from build123d import *

# Parameters (mm, degrees)
SKETCH3_R                = 3.571875
SKETCH3_R_2              = 1.5319375
SKETCH3_R_3              = 2.778125
SKETCH3_R_4              = 0.813693974
BOSS_EXTRUDE1_DEPTH      = 7.9375
BOSS_EXTRUDE2_DEPTH      = 9.525
BOSS_EXTRUDE2_DEPTH_BACK = 1.5875
SKETCH3_4_R              = 1.5319375
FILLET1_R                = 1.5875
SKETCH4_W                = 1.5875
SKETCH4_H                = 4.7625
CUT_EXTRUDE1_DEPTH       = 3.175
SKETCH5_W                = 4.7752
SKETCH5_H                = 1.5875
CUT_EXTRUDE2_DEPTH       = 3.175
FILLET2_R                = 3.571875
SKETCH6_R                = 0.4064
CUT_EXTRUDE4_DEPTH       = 0.89281
CUT_EXTRUDE6_START       = -1.5875
CUT_EXTRUDE6_DEPTH       = 1.5875
CUT_EXTRUDE7_START       = -7.9375
CUT_EXTRUDE7_DEPTH       = 1.5875
FILLET4_R                = 1.5875


with BuildPart() as part:
    # Sketch3 → Boss-Extrude1 (new body)
    # profile 1 of 12: a face of its own
    with BuildSketch(Plane.XY):
        with BuildLine():
            Line((11.069438658, 5.55625), (2.778125, 5.55625))
            ThreePointArc((2.778125, 5.55625), (4.742556026, 4.742556026), (5.55625, 2.778125))
            ThreePointArc((5.55625, 2.778125), (4.742556026, 0.813693974), (2.778125, 0))
            Line((2.778125, 0), (9.649461258, 0))
            ThreePointArc((9.649461258, 0), (10.438552252, 3.141997614), (13.44291972, 4.353851449))
            ThreePointArc((13.44291972, 4.353851449), (12.140043825, 4.7258047), (11.069438658, 5.55625))
        make_face()
    # profile 2 of 12: a face of its own
    with BuildSketch(Plane.XY):
        with Locations((13.754229109, 7.912134389)):
            Circle(SKETCH3_R)
        with Locations((13.754229109, 7.912134389)):
            Circle(SKETCH3_R_2, mode=Mode.SUBTRACT)
    # profile 3 of 12: a face of its own
    with BuildSketch(Plane.XY):
        with Locations((2.778125, 2.778125)):
            Circle(SKETCH3_R_3)
    # profile 4 of 12: a face of its own
    with BuildSketch(Plane.XY):
        with Locations((0.813693974, 4.742556026)):
            Circle(SKETCH3_R_4)
    # profile 5 of 12: a face of its own
    with BuildSketch(Plane.XY):
        with BuildLine():
            ThreePointArc((0.328789509, 4.089130022), (0.086830258, 4.376814286), (0, 4.742556026))
            Line((0, 4.742556026), (0, 2.778125))
            ThreePointArc((0, 2.778125), (0.083450745, 3.453927617), (0.328789509, 4.089130022))
        make_face()
    # profile 6 of 12: a face of its own
    with BuildSketch(Plane.XY):
        with Locations((2.778125, 2.778125)):
            Circle(SKETCH3_R_3)
    # profile 7 of 12: a face of its own
    with BuildSketch(Plane.XY):
        with Locations((0.813693974, 4.742556026)):
            Circle(SKETCH3_R_4)
    # profile 8 of 12: a face of its own
    with BuildSketch(Plane.XY):
        with Locations((0.813693974, 4.742556026)):
            Circle(SKETCH3_R_4)
    # profile 9 of 12: a face of its own
    with BuildSketch(Plane.XY):
        with Locations((2.778125, 2.778125)):
            Circle(SKETCH3_R_3)
    # profile 10 of 12: a face of its own
    with BuildSketch(Plane.XY):
        with BuildLine():
            Line((2.778125, 5.55625), (0.813693974, 5.55625))
            ThreePointArc((0.813693974, 5.55625), (1.179435714, 5.469419742), (1.467119978, 5.227460491))
            ThreePointArc((1.467119978, 5.227460491), (2.102322383, 5.472799255), (2.778125, 5.55625))
        make_face()
    # profile 11 of 12: a face of its own
    with BuildSketch(Plane.XY):
        with BuildLine():
            ThreePointArc((2.778125, 0), (0.813693974, 0.813693974), (0, 2.778125))
            Line((0, 2.778125), (0, 0))
            Line((0, 0), (2.778125, 0))
        make_face()
    # profile 12 of 12: a face of its own
    with BuildSketch(Plane.XY):
        Polygon((0, -3.175), (9.649461258, -3.175), (9.649461258, 0), (2.778125, 0), (0, 0), align=None)
    extrude(amount=BOSS_EXTRUDE1_DEPTH)

    # Sketch3_4 → Boss-Extrude2 (add, two sides: drawn at the far end of the back side and taken through both)
    with BuildSketch(Plane.XY.offset(-BOSS_EXTRUDE2_DEPTH_BACK)):
        with Locations((13.754229109, 7.912134389)):
            Circle(SKETCH3_4_R)
    extrude(amount=BOSS_EXTRUDE2_DEPTH + BOSS_EXTRUDE2_DEPTH_BACK)

    # Fillet1
    fillet1_edges = [part.edges().sort_by_distance(p)[0] for p in [
        (9.649461258, 0, 3.96875),
        (9.649461258, -3.175, 3.96875),
        (0, -3.175, 3.96875),
    ]]
    fillet(fillet1_edges, radius=FILLET1_R)

    # Sketch4 → Cut-Extrude1 (cut)
    with BuildSketch(Plane.XZ.offset(3.175)):
        with Locations((4.824730629, 3.96875)):
            Rectangle(SKETCH4_W, SKETCH4_H)
    extrude(amount=-CUT_EXTRUDE1_DEPTH, mode=Mode.SUBTRACT)

    # Sketch5 → Cut-Extrude2 (cut)
    with BuildSketch(Plane.ZY):
        with Locations((3.96875, 1.577528013)):
            Rectangle(SKETCH5_W, SKETCH5_H)
    extrude(amount=-CUT_EXTRUDE2_DEPTH, mode=Mode.SUBTRACT)

    # Fillet2
    fillet2_edges = [part.edges().sort_by_distance(p)[0] for p in [
        (11.069438658, 5.55625, 3.96875),
    ]]
    fillet(fillet2_edges, radius=FILLET2_R)

    # Sketch6 → Cut-Extrude4 (cut)
    with BuildSketch(Plane(origin=(17.326104109, 0, 0), x_dir=(0, 0, -1), z_dir=(1, 0, 0))):
        with Locations((-3.96875, 7.912134389)):
            Circle(SKETCH6_R)
        with BuildLine():
            ThreePointArc((-3.56235, 7.912134389), (-3.681381804, 7.624766193), (-3.96875, 7.505734389))
            Line((-3.96875, 7.505734389), (-3.56235, 7.505734389))
            Line((-3.56235, 7.505734389), (-3.56235, 7.912134389))
        make_face()
        with BuildLine():
            Line((-4.37515, 7.912134389), (-4.37515, 7.505734389))
            Line((-4.37515, 7.505734389), (-3.96875, 7.505734389))
            ThreePointArc((-3.96875, 7.505734389), (-4.256118196, 7.624766193), (-4.37515, 7.912134389))
        make_face()
        with BuildLine():
            Line((-4.37515, 8.318534389), (-4.37515, 7.912134389))
            ThreePointArc((-4.37515, 7.912134389), (-4.256118196, 8.199502585), (-3.96875, 8.318534389))
            Line((-3.96875, 8.318534389), (-4.37515, 8.318534389))
        make_face()
        with BuildLine():
            ThreePointArc((-3.96875, 8.318534389), (-3.681381804, 8.199502585), (-3.56235, 7.912134389))
            Line((-3.56235, 7.912134389), (-3.56235, 8.318534389))
            Line((-3.56235, 8.318534389), (-3.96875, 8.318534389))
        make_face()
    extrude(amount=-CUT_EXTRUDE4_DEPTH, mode=Mode.SUBTRACT)

    # Sketch7 → Cut-Extrude6 (cut)
    with BuildSketch(Plane.XY.offset(7.9375).offset(CUT_EXTRUDE6_START)):
        with BuildLine():
            ThreePointArc((10.234480151, 8.520129694), (14.059341963, 11.470954019), (17.326104109, 7.912134389))
            ThreePointArc((17.326104109, 7.912134389), (16.167352882, 5.278671901), (13.44291969, 4.353851452))
            ThreePointArc((13.44291969, 4.353851452), (12.109733834, 4.218149348), (10.920382704, 3.600700179))
            ThreePointArc((10.920382704, 3.600700179), (16.203542696, 3.371207904), (18.913604109, 7.912134389))
            ThreePointArc((18.913604109, 7.912134389), (12.924190998, 13.004303585), (8.861926483, 6.273682251))
            ThreePointArc((8.861926483, 6.273682251), (9.762713445, 7.265842741), (10.234480151, 8.520129694))
        make_face()
        with BuildLine():
            ThreePointArc((13.44291969, 4.353851452), (10.924260793, 5.732783489), (10.234480151, 8.520129694))
            ThreePointArc((10.234480151, 8.520129694), (9.762713445, 7.265842741), (8.861926483, 6.273682251))
            ThreePointArc((8.861926483, 6.273682251), (9.666497097, 4.764183089), (10.920382704, 3.600700179))
            ThreePointArc((10.920382704, 3.600700179), (12.109733834, 4.218149348), (13.44291969, 4.353851452))
        make_face()
    extrude(amount=CUT_EXTRUDE6_DEPTH, mode=Mode.SUBTRACT)

    # Sketch7_6 → Cut-Extrude7 (cut)
    with BuildSketch(Plane.XY.offset(7.9375).offset(CUT_EXTRUDE7_START)):
        with BuildLine():
            ThreePointArc((10.234480151, 8.520129694), (14.059341963, 11.470954019), (17.326104109, 7.912134389))
            ThreePointArc((17.326104109, 7.912134389), (16.167352882, 5.278671901), (13.44291969, 4.353851452))
            ThreePointArc((13.44291969, 4.353851452), (12.109733834, 4.218149348), (10.920382704, 3.600700179))
            ThreePointArc((10.920382704, 3.600700179), (16.203542696, 3.371207904), (18.913604109, 7.912134389))
            ThreePointArc((18.913604109, 7.912134389), (12.924190998, 13.004303585), (8.861926483, 6.273682251))
            ThreePointArc((8.861926483, 6.273682251), (9.762713445, 7.265842741), (10.234480151, 8.520129694))
        make_face()
        with BuildLine():
            ThreePointArc((13.44291969, 4.353851452), (10.924260793, 5.732783489), (10.234480151, 8.520129694))
            ThreePointArc((10.234480151, 8.520129694), (9.762713445, 7.265842741), (8.861926483, 6.273682251))
            ThreePointArc((8.861926483, 6.273682251), (9.666497097, 4.764183089), (10.920382704, 3.600700179))
            ThreePointArc((10.920382704, 3.600700179), (12.109733834, 4.218149348), (13.44291969, 4.353851452))
        make_face()
    extrude(amount=CUT_EXTRUDE7_DEPTH, mode=Mode.SUBTRACT)

    # Fillet4
    fillet4_edges = [part.edges().sort_by_distance(p)[0] for p in [
        (8.861926483, 6.273682251, 7.14375),
        (10.920382704, 3.600700179, 7.14375),
        (8.861926483, 6.273682251, 0.79375),
        (10.920382704, 3.600700179, 0.79375),
    ]]
    fillet(fillet4_edges, radius=FILLET4_R)


solid = part.part
Can you work these out from the model? Positions are in its coordinate system, mm. A direction names the side the tool comes from. Coordinates: 2 decimals unless noted, no trailing zeros. Write each loop counter-clockwise with the first axis right and the second up, starting at its lowest first coordinate (ties: lowest second). Pieces come first, ordered by that corner, then holes. Notation, with made-up numbers: (-28.75, 3) -> (-6.75, 3) arc R18 ccw to (-6.75, 14) -> close; hole circle Ø7 at (-18.75, 38.25). An arc over 180 degrees is marked (long way). Write each question's results on one line, items separated by ' | '. Start each with the question number.
Q1. We'd pull the mould along Y, two halves only. Please class faces 1 (the face through (17, 8, 4.375)), 2 (the face through (5.618, -2, 4)), 3 (the face through (0.24, 5.32, 3.91)), 4 (the face through (0.477, -2.722, 4.024)): +Y half, -Y half, draft (parallel to the pull), parting line (faces both ways), or undercut.
Q2. If I drill on probe 1 along Z at (x, y) = (2.75, 2); probe 2 along Y at (x, z) = (5.5, 1.25) (3 decimals); probe 3 along Z at (x, y) = (6.25, 5.25), over which ranges is the centre line in solid material (lowest first)?
Q3. Imagine slicing it at A-A (x = 2.5). Write out the boundary of the cut face in (y, z) (1 decimal).
Q4. I'm going to push flat-ended pins straight in: pin 1 (1.3 mm diameter, centred on y = 1.5, z = 5, fed in from -X) (3 decimals); pin 2 (0.8 mm diameter, centred on x = 2, y = 2, fed in from +Z); pin 3 (3 mm diameter, centred on x = 5, z = 3.5, fed in from +Y). Where does each tip first touch, or does it pass through?
Q5. Imagine slicing it at D-D (y = 1.5). Write out the boundary of the cut face in (x, z) (1 decimal), then the cut area to 3 significant figures.
Q6. On a 3-axis mill with a long thin cutter (end or side, diameter ignored), from which of +Z, -Z, +X, -X, +Y, -Y can I reach the whole of each face in a straight line? I mean faces 5 (the face through (2, 2, 1.581)), 6 (the face through (4, 5.556, 4)), 7 (the face through (16.433, 8, 4)), 8 (the face through (15.17, 7.33, -0.8)). Say none if no direction works.
Taken from the geometry:
1) face 1: undercut | face 2: draft | face 3: +Y half | face 4: -Y half
2) probe 1: z = 0 to 1.58, 6.36 to 7.94 | probe 2: y = -3.175 to 5.556 | probe 3: z = 0 to 7.94
3) outline: (-3.2, 0) -> (5.6, 0) -> (5.6, 7.9) -> (-3.2, 7.9) -> close; hole (0.8, 1.6) -> (2.4, 1.6) -> (2.4, 6.4) -> (0.8, 6.4) -> close
4) pin 1: stops at x = 3.175 | pin 2: stops at z = 7.94 | pin 3: stops at y = 5.56
5) outline: (0, 0) -> (9.6, 0) -> (9.6, 7.9) -> (0, 7.9) -> (0, 6.4) -> (3.2, 6.4) -> (3.2, 1.6) -> (0, 1.6) -> close | area: 61.3 mm^2
6) face 5: -X | face 6: +Z, -Z, -X, +Y | face 7: +X | face 8: -Z
